Could you check a few things on this model? Use its own coordinates, in mm. A direction names the side the tool comes from. Give positions to 0.01 mm unless a question says otherwise; leave off trailing zeros. Loops run counter-clockwise (first coordinate to the right, second up) from the corner with the lowest first, then second, coordinate; pieces in that order, holes last. Notation, with made-up numbers: (11.5, 81) -> (40.5, 81) arc R17 cw to (40.5, 88) -> close; hole circle Ø3 at (78.25, -30.5). An arc over 180 degrees is marked (long way). Write each question's results on one line, items separated by ' | '. Start each with the question number.
Q1. If I drill on line 1 along Y through (x, z) = (29, 45.5); line 2 along Y through (x, z) = (31, 43); line 3 along Z through (x, y) = (18, -17.5), over which ranges is the centre line in solid material (lowest first)?
Q2. If we section it at A-A, the plane z = 35.5: List the corners of the cut face in (x, y) for me, plus the area to 3 significant figures.
Q3. Which directions (+Z, -Z, +X, -X, +Y, -Y) give clear straight access to the entire face, cutting with the end or side of a thin tool? Please do faces 1 (the face through (9, -23, 61.571)), 2 (the face through (16.688, -1.146, 67.494)), 3 (the face through (9, -23, 58.498)).
Q4. Will these pins go through, and if not, where does the flat tip stop? P1, Ø3.5, axis at y = -23.5, z = 59.5, coming from the -X side; P2, Ø0.9, axis at x = 9, y = -22.5, coming from the -Z side; P3, Ø0.9, axis at y = -23, z = 59.5, coming from the +X side.
Q5. If we section it at B-B, the plane x = 19: List the corners of the cut face in (y, z) for me.
from build123d import *

# Parameters (mm, degrees)
F0_W     = 33.02
F0_H     = 68.58
F1_DEPTH = 20.32
F2_R     = 3.81
F3_W     = 3.073085
F3_H     = 3.073089
F4_DEPTH = 4.572


with BuildPart() as f1:
    # F0 (on Front) → F1 (new body)
    with BuildSketch(Plane.XZ):
        with Locations((16.51, 34.29)):
            Rectangle(F0_W, F0_H)
    extrude(amount=F1_DEPTH)

    # F2
    f2_edges = [f1.edges().sort_by_distance(p)[0] for p in [
        (33.02, -20.32, 34.29),
        (33.02, -10.16, 68.58),
        (16.51, -20.32, 68.58),
        (0, -20.32, 34.29),
        (16.51, -20.32, 0),
        (33.02, -10.16, 0),
        (33.02, 0, 34.29),
        (16.51, 0, 0),
        (0, 0, 34.29),
        (0, -10.16, 68.58),
        (0, -10.16, 0),
        (16.51, 0, 68.58),
    ]]
    fillet(f2_edges, radius=F2_R)

    # F3 (on face) → F4 (join)
    with BuildSketch(Plane.XZ.offset(20.32)):
        with Locations((9.438765, 60.034938)):
            Rectangle(F3_W, F3_H)
    extrude(amount=F4_DEPTH)


solid = f1.part
Final values:
1) line 1: y = -20.32 to 0 | line 2: y = -19.87 to -0.45 | line 3: z = 0.13 to 68.45
2) outline: (0, -16.51) arc R3.81 ccw to (3.81, -20.32) -> (29.21, -20.32) arc R3.81 ccw to (33.02, -16.51) -> (33.02, -3.81) arc R3.81 ccw to (29.21, 0) -> (3.81, 0) arc R3.81 ccw to (0, -3.81) -> close | area: 659 mm²
3) face 1: +Z, +X, -X, -Y | face 2: +Z, +X, -X, +Y | face 3: -Z, +X, -X, -Y
4) P1: stops at x = 7.9 | P2: stops at z = 58.5 | P3: stops at x = 10.98
5) outline: (-20.32, 3.81) arc R3.81 ccw to (-16.51, 0) -> (-3.81, 0) arc R3.81 ccw to (0, 3.81) -> (0, 64.77) arc R3.81 ccw to (-3.81, 68.58) -> (-16.51, 68.58) arc R3.81 ccw to (-20.32, 64.77) -> close
